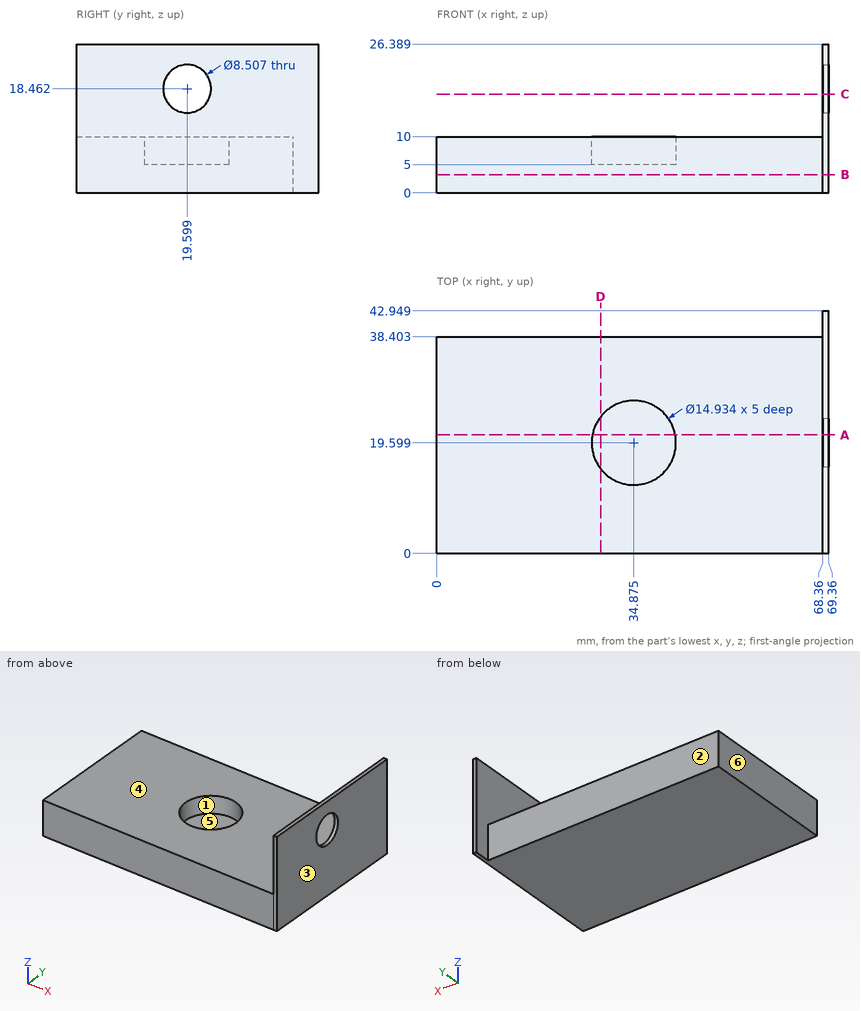
Could you check a few things on this drawing? It's one solid part, dimensions in mm from its lowest x, y, z. A direction names the side the tool comes from. Give positions to 0.01 mm unless a question says otherwise; leave off trailing zeros. Order: outer loops, then holes, each group sorted by start corner. A loop starts at its lowest first (then second) coordinate and runs counter-clockwise, first axis right, second up. Notation, with made-up numbers: (-2, 72) -> (5, 72) arc R16 cw to (5, 86) -> close; hole circle Ø7 at (41.25, -11). An arc over 180 degrees is marked (long way). Answer in a Markdown table with one row per item. Add a question column.
Item 1: I'm going to push flat-ended pins straight in: P1, Ø2, axis at x = 54, y = 35.5, coming from the +Z side; P2, Ø3, axis at x = 22.5, z = 3.5, coming from the +Y side; P3, Ø12, axis at x = 35, y = 18.5, coming from the +Z side. Where does each tip first touch, or does it pass through?
Item 2: We'd pull the mould along X, two halves only. Please class the marked faces 1, 2 and 3: pulls with the +X half, pulls with the -X half, needs draft (parallel to the pull), parting line crosses it, or undercut.
Item 3: Please list where these lines run through material, in increasing order: probe 1 along Z at (x, y) = (21.5, 10); probe 2 along X at (y, z) = (37, 23.25); probe 3 along Y at (x, z) = (36, 3.5).
Item 4: Imagine slicing it at B-B (z = 3.25). List the corners of the cut face in (x, y) for me.
Item 5: Imagine slicing it at D-D (x = 29). List the corners of the cut face in (y, z) for me, and give its area (3 significant figures).
Item 6: For the marked faces 4, 5 and 6, which set-ups out of +Z, -Z, +X, -X, +Y, -Y let a thin tool reach every point of the face, with its end or its side?
Item 7: Imagine slicing it at C-C (z = 17.5). List the corners of the cut face in (x, y) for me (1 decimal).
Item 8: Imagine slicing it at A-A (y = 21). List the corners of the cut face in (x, z) for me.
Result:
| question | item | result |
|---|---|---|
| 1 | P1 | z = 10 |
| 1 | P2 | y = 38.4 |
| 1 | P3 | z = 5 |
| 2 | face 1 | undercut |
| 2 | face 2 | needs draft |
| 2 | face 3 | pulls with the +X half |
| 3 | probe 1 | 0 to 10 |
| 3 | probe 2 | 68.36 to 69.36 |
| 3 | probe 3 | 0 to 38.4 |
| 4 | outline | (0, 0) -> (69.36, 0) -> (69.36, 42.95) -> (68.36, 42.95) -> (68.36, 38.4) -> (0, 38.4) -> close |
| 5 | outline | (0, 0) -> (38.4, 0) -> (38.4, 10) -> (24.21, 10) -> (24.21, 5) -> (14.99, 5) -> (14.99, 10) -> (0, 10) -> close |
| 5 | area | 338 mm2 |
| 6 | face 4 | +Z, -X, +Y, -Y |
| 6 | face 5 | +Z |
| 6 | face 6 | +Z, -Z, -X, +Y, -Y |
| 7 | outline | (68.4, 0) -> (69.4, 0) -> (69.4, 15.5) -> (68.4, 15.5) -> close; (68.4, 23.7) -> (69.4, 23.7) -> (69.4, 42.9) -> (68.4, 42.9) -> close |
| 8 | outline | (0, 0) -> (69.36, 0) -> (69.36, 14.45) -> (68.36, 14.45) -> (68.36, 10) -> (42.21, 10) -> (42.21, 5) -> (27.54, 5) -> (27.54, 10) -> (0, 10) -> close; (68.36, 22.48) -> (69.36, 22.48) -> (69.36, 26.39) -> (68.36, 26.39) -> close |
